```python
from build123d import *

# Parameters (mm, degrees)
SKETCH_1_W               = 20
SKETCH_1_H               = 20
SKETCH_1_W_2             = 16
SKETCH_1_H_2             = 16
EXTRUDE_1_DEPTH          = 970
SKETCH_2_R               = 4.05
CUT_EXTRUDE_1_DEPTH      = 970
SKETCH_4_W               = 21.376287738
SKETCH_4_H               = 29.089038522
CUT_EXTRUDE_3_DEPTH      = 50
SKETCH_6_R               = 1
CUT_EXTRUDE_5_DEPTH      = 10
M4X0_7_1_D               = 3.3
M4X0_7_1_DEPTH           = 5
M4X0_7_1_TIP             = 0.991420021
SKETCH_10_R              = 1
CUT_EXTRUDE_6_DEPTH      = 5
M4X0_7_4_D               = 3.3
M4X0_7_4_DEPTH           = 5
M4X0_7_4_TIP             = 0.991420021
M4X0_7_4_ON_FACE_2_D     = 3.3
M4X0_7_4_ON_FACE_2_DEPTH = 5
M4X0_7_4_ON_FACE_2_TIP   = 0.991420021
SKETCH_12_R              = 1
CUT_EXTRUDE_7_DEPTH      = 5
M4X0_7_5_D               = 3.3
M4X0_7_5_DEPTH           = 9
M4X0_7_5_TIP             = 0.991420021
M4X0_7_5_ON_FACE_2_D     = 3.3
M4X0_7_5_ON_FACE_2_DEPTH = 9
M4X0_7_5_ON_FACE_2_TIP   = 0.991420021


with BuildPart() as part:
    # ｽｹｯﾁ1 → ﾎﾞｽ - 押し出し1 (new body)
    with BuildSketch(Plane.XY):
        Rectangle(SKETCH_1_W, SKETCH_1_H)
        Rectangle(SKETCH_1_W_2, SKETCH_1_H_2, mode=Mode.SUBTRACT)
    extrude(amount=EXTRUDE_1_DEPTH)

    # ｽｹｯﾁ2 → ｶｯﾄ - 押し出し1 (cut)
    with BuildSketch(Plane(origin=(10, 0, 0), x_dir=(0, 0, -1), z_dir=(1, 0, 0))):
        with Locations((-50, 0)):
            Circle(SKETCH_2_R)
    extrude(amount=-CUT_EXTRUDE_1_DEPTH, mode=Mode.SUBTRACT)

    # ｽｹｯﾁ4 → ｶｯﾄ - 押し出し3 (cut)
    with BuildSketch(Plane.XY.offset(970)):
        Rectangle(SKETCH_4_W, SKETCH_4_H)
    extrude(amount=-CUT_EXTRUDE_3_DEPTH, mode=Mode.SUBTRACT)

    # ｽｹｯﾁ6 → ｶｯﾄ - 押し出し5 (cut)
    with BuildSketch(Plane.XZ.offset(10)):
        with Locations((0, 30)):
            Circle(SKETCH_6_R)
        with Locations((0, 50)):
            Circle(SKETCH_6_R)
    extrude(amount=-CUT_EXTRUDE_5_DEPTH, mode=Mode.SUBTRACT)

    # M4x0.7 ねじ穴1
    with Locations(Plane(origin=(0, -10, 30), x_dir=(0, 0, -1), z_dir=(0, -1, 0))):
        with Locations((0, 0), (-20, 0)):
            Hole(M4X0_7_1_D / 2, depth=M4X0_7_1_DEPTH)
            with Locations((0, 0, -(M4X0_7_1_DEPTH + M4X0_7_1_TIP / 2))):  # 118° drill point
                Cone(0, M4X0_7_1_D / 2, M4X0_7_1_TIP, mode=Mode.SUBTRACT)

    # ｽｹｯﾁ10 → ｶｯﾄ - 押し出し6 (cut)
    with BuildSketch(Plane(origin=(0, -10, 0), x_dir=(-1, 0, 0), z_dir=(0, -1, 0))):
        with Locations((0, -670)):
            Circle(SKETCH_10_R)
        with Locations((0, -650)):
            Circle(SKETCH_10_R)
    extrude(amount=-CUT_EXTRUDE_6_DEPTH, mode=Mode.SUBTRACT)

    # M4x0.7 ねじ穴4
    with Locations(Plane(origin=(0, -10, 650), x_dir=(0, 0, -1), z_dir=(0, -1, 0))):
        with Locations((0, 0)):
            Hole(M4X0_7_4_D / 2, depth=M4X0_7_4_DEPTH)
            with Locations((0, 0, -(M4X0_7_4_DEPTH + M4X0_7_4_TIP / 2))):  # 118° drill point
                Cone(0, M4X0_7_4_D / 2, M4X0_7_4_TIP, mode=Mode.SUBTRACT)

    # M4x0.7 ねじ穴4 on face 2
    with Locations(Plane(origin=(0, -8, 670), x_dir=(0, 0, -1), z_dir=(0, -1, 0))):
        with Locations((0, 0)):
            Hole(M4X0_7_4_ON_FACE_2_D / 2, depth=M4X0_7_4_ON_FACE_2_DEPTH)
            with Locations((0, 0, -(M4X0_7_4_ON_FACE_2_DEPTH + M4X0_7_4_ON_FACE_2_TIP / 2))):  # 118° drill point
                Cone(0, M4X0_7_4_ON_FACE_2_D / 2, M4X0_7_4_ON_FACE_2_TIP, mode=Mode.SUBTRACT)

    # ｽｹｯﾁ12 → ｶｯﾄ - 押し出し7 (cut)
    with BuildSketch(Plane.ZY.offset(10)):
        with Locations((710, 0)):
            Circle(SKETCH_12_R)
        with Locations((730, 0)):
            Circle(SKETCH_12_R)
        with Locations((40, 0)):
            Circle(SKETCH_12_R)
    extrude(amount=-CUT_EXTRUDE_7_DEPTH, mode=Mode.SUBTRACT)

    # M4x0.7 ねじ穴5
    with Locations(Plane(origin=(-10, 0, 730), x_dir=(0, 0, -1), z_dir=(-1, 0, 0))):
        with Locations((0, 0), (20, 0)):
            Hole(M4X0_7_5_D / 2, depth=M4X0_7_5_DEPTH)
            with Locations((0, 0, -(M4X0_7_5_DEPTH + M4X0_7_5_TIP / 2))):  # 118° drill point
                Cone(0, M4X0_7_5_D / 2, M4X0_7_5_TIP, mode=Mode.SUBTRACT)

    # M4x0.7 ねじ穴5 on face 2
    with Locations(Plane(origin=(-8, 0, 40), x_dir=(0, 0, -1), z_dir=(-1, 0, 0))):
        with Locations((0, 0)):
            Hole(M4X0_7_5_ON_FACE_2_D / 2, depth=M4X0_7_5_ON_FACE_2_DEPTH)
            with Locations((0, 0, -(M4X0_7_5_ON_FACE_2_DEPTH + M4X0_7_5_ON_FACE_2_TIP / 2))):  # 118° drill point
                Cone(0, M4X0_7_5_ON_FACE_2_D / 2, M4X0_7_5_ON_FACE_2_TIP, mode=Mode.SUBTRACT)


solid = part.part
```
Build history of the part. All positions in model axes, mm. A direction names the side the tool comes from. Coordinates: 2 decimals unless noted, no trailing zeros. Order: outer loops, then holes, each group sorted by start corner. A loop starts at its lowest first (then second) coordinate and runs counter-clockwise, first axis right, second up. Notation, with made-up numbers: (23, -29) -> (69, -29) arc R36 ccw to (69, 5) -> close; hole circle Ø11 at (-32, 59.25). An arc over 180 degrees is marked (long way). Answer in a Markdown table with one row per item. Add a question column.
Q1. Wall check: line 1 along X through (y, z) = (-5, 743.5); line 2 along X through (y, z) = (-9.5, 50). Give the ranges that are in metal, low to high. Write a range as [from, to].
Q2. Drop flat-ended pins along their axis: pin 1 (2 mm diameter, centred on x = 0, z = 50, fed in from -Y); pin 2 (3 mm diameter, centred on y = 0, z = 710, fed in from -X); pin 3 (7.5 mm diameter, centred on y = 0, z = 50, fed in from -X). Give the stop position or say it passes through.
Q3. Band-saw the part on A-A, the plane z = 237.5. List the corners of the cut face in (x, y).
Q4. Which spindle directions (+Z, -Z, +X, -X, +Y, -Y) get a long thin tool onto all of the face, cutting with end or side? Do faces 4 (the face through (0, 8, 454)), 5 (the face through (-9, 0, 920)). Say none if no direction does.
Q5. Mould opens along Y. For faces 1 (the face through (0, 10, 454)), 2 (the face through (-8, 0, 454)), 3 (the face through (10, 0, 454)) say: +Y half, -Y half, draft (parallel to the pull), parting line (faces both ways), or undercut.
Answers follow:
| question | item | result |
|---|---|---|
| 1 | line 1 | [-10, -8], [8, 10] |
| 1 | line 2 | [-10, -1.65], [1.65, 10] |
| 2 | pin 1 | y = 8 |
| 2 | pin 2 | x = 8 |
| 2 | pin 3 | through |
| 3 | outline | (-10, -10) -> (10, -10) -> (10, 10) -> (-10, 10) -> close; hole (-8, -8) -> (8, -8) -> (8, 8) -> (-8, 8) -> close |
| 4 | face 4 | +Z, -Z |
| 4 | face 5 | +Z, +X, -X, +Y, -Y |
| 5 | face 1 | +Y half |
| 5 | face 2 | undercut |
| 5 | face 3 | draft |
